Autodesk Inventor part; units mm, degrees
ref_plane "YZ Plane" through (0, 0, 0) normal (1, 0, 0) x (0, 1, 0)
ref_plane "XZ Plane" through (0, 0, 0) normal (0, 1, 0) x (-1, 0, 0)
ref_plane "XY Plane" through (0, 0, 0) normal (0, 0, 1) x (1, 0, 0)
sketch "Sketch1" plane through (0, 0, 0) normal (0, 0, 1) x (1, 0, 0)
  line L0 (27.5881, 10.0556) -> (27.8558, 9.3368) construction
  line L1 (27.8558, 9.3368) -> (21.3609, 5.6433) construction
  arc A0 (21.3609, 5.6433) -> (19.6075, 2.6357) centre (22.5174, 2.9541) ccw construction
  arc A1 (19.529, -3.031) -> (19.6075, 2.6357) centre (-6.8308, 0.1684) ccw construction
  arc A2 (19.529, -3.031) -> (21.1242, -6.2153) centre (22.4904, -3.5391) ccw construction
  line L2 (27.6234, -9.961) -> (21.1242, -6.2153) construction
  line L3 (27.6234, -9.961) -> (27.3665, -10.6837) construction
  line L4 (14.515, -25.5221) -> (13.8537, -25.9105)
  circle A3 centre (0, 0) radius 7.9375
  circle A4 centre (0, 0) radius 29.3688
  point P0 (27.495, -10.3223)
  point P1 (27.722, 9.6962)
  dimension "d0" = 15.875
  dimension "d1" = 26.5532
  dimension "d2" = 58.7375
extrude "Extrusion1" add sketch "Sketch1" along normal blind 2.794
sketch "Sketch2" plane through (0, 0, 2.794) normal (0, 0, 1) x (1, 0, 0)
  line L0 (-9.6157, 27.75) -> (-5.4166, 20.4769)
  arc A0 (-5.4166, 20.4769) -> (-2.286, 18.9123) centre (-2.667, 22.0644) ccw
  arc A1 (2.286, 18.9123) -> (5.4166, 20.4769) centre (2.667, 22.0644) ccw
  line L1 (9.6157, 27.75) -> (5.4166, 20.4769)
  line L2 (0, 0) -> (0, 29.4775) construction
  arc A2 (2.286, 18.9123) -> (-2.286, 18.9123) centre (0, 0) ccw
  circle A3 centre (0, 0) radius 29.3687
  dimension "d8" = 60
  dimension "d9" = 19.05
  dimension "d10" = 3.175
  dimension "d11" = 5.334
extrude "Extrusion2" cut sketch "Sketch2" against normal through all contours A3 L1 A1 A2 A0 L0 picked at (0.2545, 25.8031)
pattern_circular "Circular Pattern1" count 9 over 360 about axis through (0, 0, 0) along (0, 0, 1) of "Extrusion2"
properties part number "ROLLER,5"
Verification items for the finished model (mm, model axes). A direction names the side the tool comes from. Give positions to 0.01 mm unless a question says otherwise; leave off trailing zeros. Write each loop counter-clockwise with the first axis right and the second up, starting at its lowest first coordinate (ties: lowest second). Pieces come first, ordered by that corner, then holes. Notation, with made-up numbers: (-3, -29) - (43, -29) arc R30 ccw to (43, 4) - close; hole circle Ø1 at (79.25, 42). An arc over 180 degrees is marked (long way). Put each result on its own line as item: value.
Q1. Scan lines: probe 1 along Y at (x, z) = (0, 1.2); probe 2 along X at (y, z) = (-19, 0.45); probe 3 along Y at (x, z) = (-17.5, 0.15). Record each from-to range of solid material in increasing order. Write a range as from..to.
Result:
probe 1: -29.37..-7.94, 7.94..19.05
probe 2: -17.38..-14.01, -3.29..3.29, 14.01..17.38
probe 3: -21.93..-19.22, -7.53..12.27
Q2. Mould release check, pull along X, two halves, no side actions. Record for faces 1 (the face through (-9.752, 23.361, 1.417)), 2 (the face through (-12.22, 14.614, 1.417)), 3 (the face through (-4.4, -7, 2.794)): released by +X, released by -X, zero draft, split by the parting line, or undercut.
Result:
face 1: released by -X
face 2: undercut
face 3: zero draft
Q3. Section check B-B on x = -13. Record the cut outline in (y, z), and give its area (3 significant figures).
Result:
outline: (-18.15, 0) - (13.92, 0) - (13.92, 2.79) - (-18.15, 2.79) - close
area: 89.6 mm2
Q4. Section check A-A on y = 0. Record the cut outline in (x, z), and give its area (3 significant figures).
Result:
outline: (-19.25, 0) - (-7.94, 0) - (-7.94, 2.79) - (-19.25, 2.79) - close; (7.94, 0) - (19.25, 0) - (19.25, 2.79) - (7.94, 2.79) - close
area: 63.2 mm2
Q5. Section check C-C on y = -10. Record the cut outline in (x, z), and give its area (3 significant figures).
Result:
outline: (-16.21, 0) - (16.21, 0) - (16.21, 2.79) - (-16.21, 2.79) - close
area: 90.6 mm2
Q6. Depth check by flat-ended pin: P1, Ø6, axis at x = -14.5, y = -8, coming from the -Z side; P2, Ø1, axis at y = 4, z = 0.5, coming from the +X side. Enter the tip coordinate at first touch or a pass-through.
Result:
P1: z = 0
P2: x = 18.73
Q7. Set-up check for faces 4 (the face through (21.31, 13.66, 1.42)), 5 (the face through (19.63, -0.67, 1.42)), 6 (the face through (-16.51, -9.5, 1.42)): record each of +Z, -Z, +X, -X, +Y, -Y from which the full face is reachable in a straight line by a thin tool's end or side.
Result:
face 4: +Z, -Z, +Y
face 5: +Z, -Z, +X
face 6: +Z, -Z, -X
